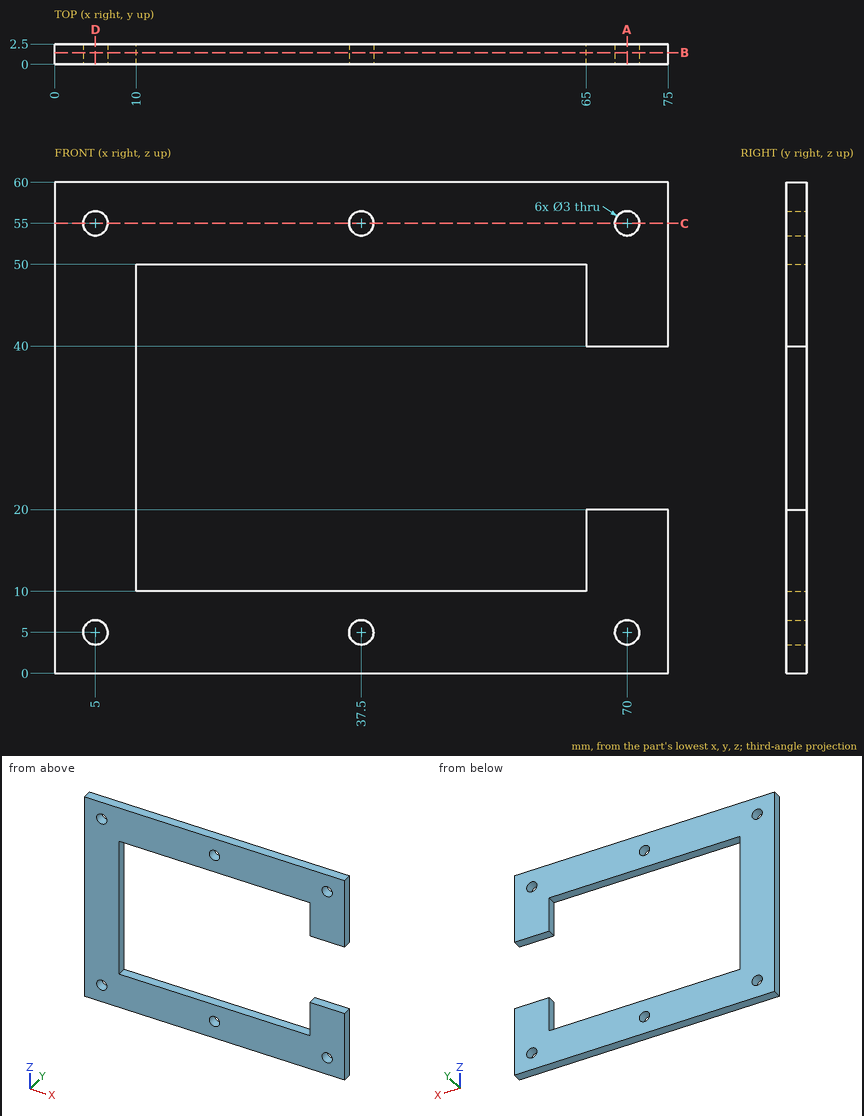
Input: dimensioned drawing with shaded views. Units: mm. Origin: part minimum x, y, z. Give positions to 0.01 mm unless a question says otherwise; leave off trailing zeros. Write each loop counter-clockwise with the first axis right and the second up, starting at its lowest first coordinate (ties: lowest second). Pieces come first, ordered by that corner, then holes.
Q1. Material intervals for probe 1 along X at (y, z) = (1.6, 5); probe 2 along Z at (x, y) = (5, 1.1); probe 3 along Z at (x, y) = (70, 0.6), sorted ascending.
Q2. Section B-B, the plane y = 1.45. Output: boundary loops of the cut face in (x, z).
Q3. Section C-C, the plane z = 55. Output: boundary loops of the cut face in (x, y).
Q4. Section A-A, the plane x = 70. Output: boundary loops of the cut face in (y, z).
Q5. Section D-D, the plane x = 5. Output: boundary loops of the cut face in (y, z), plus the area to 3 significant figures.
Q6. First-contact query: P1, Ø2.5, axis at x = 70, z = 5, coming from the +Y side. Flat tip, straight axial feed; report the tip coordinate or a pass-through.
Filled in:
1. probe 1: x = 0 to 3.5, 6.5 to 36, 39 to 68.5, 71.5 to 75
1. probe 2: z = 0 to 3.5, 6.5 to 53.5, 56.5 to 60
1. probe 3: z = 0 to 3.5, 6.5 to 20, 40 to 53.5, 56.5 to 60
2. outline: (0, 0) - (75, 0) - (75, 20) - (65, 20) - (65, 10) - (10, 10) - (10, 50) - (65, 50) - (65, 40) - (75, 40) - (75, 60) - (0, 60) - close; hole circle Ø3 at (5, 5); hole circle Ø3 at (5, 55); hole circle Ø3 at (37.5, 5); hole circle Ø3 at (37.5, 55); hole circle Ø3 at (70, 5); hole circle Ø3 at (70, 55)
3. outline: (0, 0) - (3.5, 0) - (3.5, 2.5) - (0, 2.5) - close; (6.5, 0) - (36, 0) - (36, 2.5) - (6.5, 2.5) - close; (39, 0) - (68.5, 0) - (68.5, 2.5) - (39, 2.5) - close; (71.5, 0) - (75, 0) - (75, 2.5) - (71.5, 2.5) - close
4. outline: (0, 0) - (2.5, 0) - (2.5, 3.5) - (0, 3.5) - close; (0, 6.5) - (2.5, 6.5) - (2.5, 20) - (0, 20) - close; (0, 40) - (2.5, 40) - (2.5, 53.5) - (0, 53.5) - close; (0, 56.5) - (2.5, 56.5) - (2.5, 60) - (0, 60) - close
5. outline: (0, 0) - (2.5, 0) - (2.5, 3.5) - (0, 3.5) - close; (0, 6.5) - (2.5, 6.5) - (2.5, 53.5) - (0, 53.5) - close; (0, 56.5) - (2.5, 56.5) - (2.5, 60) - (0, 60) - close
5. area: 135 mm2
6. P1: passes through
